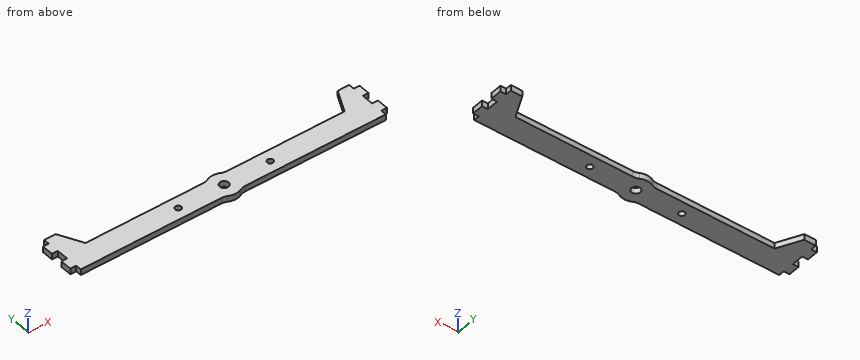
```python
from build123d import *

# Parameters (mm, degrees)
BOSS_EXTRUDE1_DEPTH      = 6.35
V_0_377_DIAMETER_HOLE1_D = 9.5758
FILLET2_R                = 12.7
F_0_257_DIAMETER_HOLE1_D = 6.5278


with BuildPart() as part:
    # Sketch1 → Boss-Extrude1 (new body)
    with BuildSketch(Plane.XY):
        with BuildLine():
            Line((-168.275, -6.35), (-168.275, -12.7))
            Line((-168.275, -12.7), (-142.875, -12.7))
            Line((-142.875, -12.7), (-9.525, -12.7))
            ThreePointArc((-9.525, -12.7), (0, -15.875), (9.525, -12.7))
            Line((9.525, -12.7), (142.875, -12.7))
            Line((142.875, -12.7), (168.275, -12.7))
            Line((168.275, -12.7), (168.275, -6.35))
            Line((168.275, -6.35), (174.625, -6.35))
            Line((174.625, -6.35), (174.625, 6.15))
            Line((174.625, 6.15), (168.275, 6.15))
            Line((168.275, 6.15), (168.275, 12.7))
            Line((168.275, 12.7), (168.275, 19.25))
            Line((168.275, 19.25), (174.625, 19.25))
            Line((174.625, 19.25), (174.625, 31.75))
            Line((174.625, 31.75), (168.275, 31.75))
            Line((168.275, 31.75), (168.275, 38.1))
            Line((168.275, 38.1), (155.575, 38.1))
            Line((155.575, 38.1), (142.875, 12.7))
            Line((142.875, 12.7), (9.525, 12.7))
            ThreePointArc((9.525, 12.7), (0, 15.875), (-9.525, 12.7))
            Line((-9.525, 12.7), (-142.875, 12.7))
            Line((-142.875, 12.7), (-155.575, 38.1))
            Line((-155.575, 38.1), (-168.275, 38.1))
            Line((-168.275, 38.1), (-168.275, 31.75))
            Line((-168.275, 31.75), (-174.625, 31.75))
            Line((-174.625, 31.75), (-174.625, 19.25))
            Line((-174.625, 19.25), (-168.275, 19.25))
            Line((-168.275, 19.25), (-168.275, 12.7))
            Line((-168.275, 12.7), (-168.275, 6.15))
            Line((-168.275, 6.15), (-174.625, 6.15))
            Line((-174.625, 6.15), (-174.625, -6.35))
            Line((-174.625, -6.35), (-168.275, -6.35))
        make_face()
    extrude(amount=BOSS_EXTRUDE1_DEPTH)

    # V (0.377) Diameter Hole1 (through all)
    with Locations(Plane.XY.offset(6.35)):
        with Locations((0, 0)):
            Hole(V_0_377_DIAMETER_HOLE1_D / 2)

    # Fillet2
    fillet2_edges = [part.edges().sort_by_distance(p)[0] for p in [
        (-9.525, 12.7, 3.175),
        (9.525, 12.7, 3.175),
        (9.525, -12.7, 3.175),
        (-9.525, -12.7, 3.175),
    ]]
    fillet(fillet2_edges, radius=FILLET2_R)

    # F (0.257) Diameter Hole1 (through all)
    with Locations(Plane.XY.offset(6.35)):
        with Locations((-50.8, -0.1), (50.8, -0.1)):
            Hole(F_0_257_DIAMETER_HOLE1_D / 2)


solid = part.part
```
Geometry check sheet. Reference: the model listing, model coordinates, mm. Give positions to 0.01 mm unless a question says otherwise; leave off trailing zeros. Write each loop counter-clockwise with the first axis right and the second up, starting at its lowest first coordinate (ties: lowest second). Pieces come first, ordered by that corner, then holes.
1) Gauge pin test, flat ends, axial feed: pin 1 (3 mm diameter, centred on x = -86.5, z = 1.5, fed in from +Y); pin 2 (3 mm diameter, centred on x = 172.5, z = 2, fed in from -Y); pin 3 (1.9 mm diameter, centred on x = -172, z = 2, fed in from +Y). Record the tip position at first contact, or that the pin passes through.
2) Section check B-B, the plane x = 0. Record the boundary of the cut face in (y, z) (3 decimals).
3) Section check C-C, the plane z = 3.5. State how many separate pieces and enclosed holes the cut face has, and give its area (3 significant figures).
4) Section check D-D, the plane x = 83. Record the boundary of the cut face in (y, z), and give its area (3 significant figures).
5) Material ranges on L1, parallel to X at y = -0.5, z = 1.5 (3 decimals); L2, parallel to Y at x = -50.8, z = 4.5; L3, parallel to Y at x = 115.5, z = 4, recorded low to high.
6) Section check A-A, the plane x = -50.8. Record the boundary of the cut face in (y, z), and give its area (3 significant figures).
Computed:
1. pin 1: stops at y = 12.7
1. pin 2: stops at y = -6.35
1. pin 3: stops at y = 31.75
2. outline: (-15.875, 0) - (-4.788, 0) - (-4.788, 6.35) - (-15.875, 6.35) - close; (4.788, 0) - (15.875, 0) - (15.875, 6.35) - (4.788, 6.35) - close
3. separate pieces: 1
3. enclosed holes: 3
3. area: 9,780 mm2
4. outline: (-12.7, 0) - (12.7, 0) - (12.7, 6.35) - (-12.7, 6.35) - close
4. area: 161 mm2
5. L1: x = -174.625 to -54.039, -47.561 to -4.762, 4.762 to 47.561, 54.039 to 174.625
5. L2: y = -12.7 to -3.36, 3.16 to 12.7
5. L3: y = -12.7 to 12.7
6. outline: (-12.7, 0) - (-3.36, 0) - (-3.36, 6.35) - (-12.7, 6.35) - close; (3.16, 0) - (12.7, 0) - (12.7, 6.35) - (3.16, 6.35) - close
6. area: 120 mm2
